```python
from build123d import *

# Parameters (mm, degrees)
F0_R     = 30
F1_DEPTH = 40
F3_DEPTH = 40


with BuildPart() as f1:
    # F0 (on Top) → F1 (new body, symmetric)
    with BuildSketch(Plane.XY):
        Circle(F0_R)
    extrude(amount=F1_DEPTH, both=True)

    # F2 (on face) → F3 (cut)
    with BuildSketch(Plane.XY.offset(40)):
        with BuildLine():
            Line((-28.284271, 10), (28.284271, 10))
            ThreePointArc((28.284271, 10), (0, 30), (-28.284271, 10))
        make_face()
        with BuildLine():
            ThreePointArc((-28.284271, -10), (0, -30), (28.284271, -10))
            Line((28.284271, -10), (-28.284271, -10))
        make_face()
    extrude(amount=-F3_DEPTH, mode=Mode.SUBTRACT)


solid = f1.part
```
Input: part model. Units: mm. Frame: model coordinates. A direction names the side the tool comes from. Give positions to 0.01 mm unless a question says otherwise; leave off trailing zeros. Order: outer loops, then holes, each group sorted by start corner. A loop starts at its lowest first (then second) coordinate and runs counter-clockwise, first axis right, second up.
1. Section D-D on y = 9. Return the cut outline in (x, z).
Derived:
outline: (-28.62, -40) - (28.62, -40) - (28.62, 40) - (-28.62, 40) - close
2. Material intervals for L1, parallel to Y at x = -10, z = 2; L2, parallel to Z at x = 16, y = 21; L3, parallel to Y at x = -22.5, z = -21, sorted ascending.
Derived:
L1: y = -10 to 10
L2: z = -40 to 0
L3: y = -19.84 to 19.84
3. Section B-B on z = -24. Return the cut outline in (x, y), and give its area (3 significant figures).
Derived:
outline: circle Ø60 at (0, 0)
area: 2,830 mm2
4. Section A-A on x = 0. Return the cut outline in (y, z).
Derived:
outline: (-30, -40) - (30, -40) - (30, 0) - (10, 0) - (10, 40) - (-10, 40) - (-10, 0) - (-30, 0) - close
5. Section C-C on x = 15. Return the cut outline in (y, z).
Derived:
outline: (-25.98, -40) - (25.98, -40) - (25.98, 0) - (10, 0) - (10, 40) - (-10, 40) - (-10, 0) - (-25.98, 0) - close
6. Pin query (flat end, axial travel): pin 1 (5 mm diameter, centred on y = -13, z = -15, fed in from -X); pin 2 (10 mm diameter, centred on x = 5, y = 19.5, fed in from +Z); pin 3 (8 mm diameter, centred on y = -8, z = -20, fed in from +X). Return the tip coordinate at first contact, or that it passes through.
Derived:
pin 1: stops at x = -28.1
pin 2: stops at z = 0
pin 3: stops at x = 29.73
7. Reachability of faces 1 (the flat face through (0, 18, 0)), 2 (the flat face through (0, -18, 0)), 3 (the flat face through (0, 0, -40)) from +Z, -Z, +X, -X, +Y, -Y: full face, straight path, thin tool, end or side. Return the list, or none.
Derived:
face 1: +Z, +X, -X, +Y
face 2: +Z, +X, -X, -Y
face 3: -Z, +X, -X, +Y, -Y
